Autodesk Fusion 360 part; units mm, degrees
sketch "Sketch1" plane through (0, 0, 0) normal (0, 1, 0) x (1, 0, 0)
  circle A0 centre (0, 0) radius 60
  dimension "d1" = 120
extrude "Extrude1" add sketch "Sketch1" along normal blind 10
sketch "Sketch2" plane through (0, 10, 0) normal (0, 1, 0) x (-1, 0, 0)
  circle A0 centre (0, 0) radius 60
  circle A1 centre (0, 0) radius 57.4
  dimension "d4" = 114.8
extrude "Extrude2" add sketch "Sketch2" along normal blind 5.3 contours A1
sketch "Sketch3" plane through (0, 15.3, 0) normal (0, 1, 0) x (-1, 0, 0)
  circle A0 centre (0, 0) radius 57.4
  circle A1 centre (0, 0) radius 60
  dimension "d7" = 120
extrude "Extrude3" add sketch "Sketch3" along normal blind 5 contours A0 | A1
sketch "Sketch4" plane through (0, 20.3, 0) normal (0, 1, 0) x (-1, 0, 0)
  circle A0 centre (0, 0) radius 60
  circle A1 centre (0, 0) radius 57.4
  dimension "d10" = 114.8
extrude "Extrude4" add sketch "Sketch4" along normal blind 5.3 contours A1
sketch "Sketch5" plane through (0, 25.6, 0) normal (0, 1, 0) x (-1, 0, 0)
  circle A0 centre (0, 0) radius 57.4
  circle A1 centre (0, 0) radius 60
  dimension "d13" = 120
extrude "Extrude5" add sketch "Sketch5" along normal blind 10 contours A0 | A1
sketch "Sketch7" plane through (0, 0, 0) normal (0, -1, 0) x (1, 0, 0)
  circle A0 centre (0, 0) radius 60
  circle A1 centre (0, 0) radius 30
  dimension "d22" = 60
extrude "Extrude7" cut sketch "Sketch7" against normal blind 10 contours A1
chamfer "Chamfer1" distance 0.5 angle 45 1 edges at (55.9396, 20.3, -21.6969)
chamfer "Chamfer2" distance 0.5 angle 45 3 edges at (55.9396, 25.6, -21.6969) (55.9396, 15.3, -21.6969) (-55.9396, 10, 21.6969)
Geometry: final body of the model. Coordinates: model frame, mm. A direction names the side the tool comes from. Coordinates: 2 decimals unless noted, no trailing zeros. Order: outer loops, then holes, each group sorted by start corner. A loop starts at its lowest first (then second) coordinate and runs counter-clockwise, first axis right, second up. Notation, with made-up numbers: (-9.75, -8) -> (16.25, -8) arc R17 ccw to (16.25, -2) -> close; hole circle Ø3 at (64.25, -33). An arc over 180 degrees is marked (long way). Write each question's results on one line, items separated by ' | '. Start each with the question number.
1) Cut plane D-D, the plane y = 29.5. Output: boundary loops of the cut face in (x, z), and give its area (3 significant figures).
2) First-contact query: pin 1 (6 mm diameter, centred on x = 24.5, z = 8.5, fed in from -Y); pin 2 (12 mm diameter, centred on x = 8.5, y = 26.5, fed in from -Z); pin 3 (8 mm diameter, centred on y = 13.5, z = 40, fed in from -X). Flat tips, straight axial feed; report the tip coordinate or a pass-through.
3) Cut plane C-C, the plane y = 11.5. Output: boundary loops of the cut face in (x, z).
4) Material intervals for line 1 along Z through (x, y) = (0, 4); line 2 along Y through (x, z) = (16.5, 4.5); line 3 along Z through (x, y) = (-53, 19), sorted ascending.
5) Mould query, pull axis Z, two halves, no side actions, for faces 1 (the flat face through (31, 25.6, 49)), 2 (the cylindrical face through (-29.97, 4.93, 1.32)), 3 (the cylindrical face through (-30.86, 12.61, -48.4)). Classes: released by +Z, released by -Z, zero draft, split by the parting line, or undercut.
6) Set-up query: faces 4 (the cylindrical face through (59.94, 17.77, -2.64)), 5 (the flat face through (0, 10, 0)), 6 (the flat face through (31, 20.3, 49)). Return all of +Z, -Z, +X, -X, +Y, -Y with unobstructed straight access to the full face (end or side cutting, diameter ignored); none if empty.
Checks:
1) outline: circle Ø120 at (0, 0) | area: 11,300 mm^2
2) pin 1: y = 10 | pin 2: z = -59.95 | pin 3: x = -47.45
3) outline: circle Ø114.8 at (0, 0)
4) line 1: -60 to -30, 30 to 60 | line 2: 10 to 35.6 | line 3: -28.12 to 28.12
5) face 1: zero draft | face 2: undercut | face 3: split by the parting line
6) face 4: +Y, -Y | face 5: -Y | face 6: none
